Could you check a few things on this model? Use its own coordinates, in mm. A direction names the side the tool comes from. Round coordinates to 2 decimals unless told otherwise and drop trailing zeros. One line per question, with ' | ' between items.
```python
from build123d import *

# Parameters (mm, degrees)
BOSS_EXTRUDE1_DEPTH = 80


with BuildPart() as part:
    # Sketch1 → Boss-Extrude1 (new body)
    with BuildSketch(Plane.XY):
        Polygon((0, 0), (61.257678877, 0), (59.423406602, 35), (58.423406602, 35), (56.851173223, 5), (55.851173223, 5), (54.278939845, 35), (53.278939845, 35), (51.706706466, 5), (50.706706466, 5), (49.134473088, 35), (48.134473088, 35), (46.562239709, 5), (45.562239709, 5), (43.990006331, 35), (42.990006331, 35), (41.417772952, 5), (40.417772952, 5), (38.845539574, 35), (37.845539574, 35), (36.273306195, 5), (35.273306195, 5), (33.701072817, 35), (32.701072817, 35), (31.128839438, 5), (30.128839438, 5), (28.55660606, 35), (27.55660606, 35), (25.984372681, 5), (24.984372681, 5), (23.412139303, 35), (22.412139303, 35), (20.839905924, 5), (19.839905924, 5), (18.267672546, 35), (17.267672546, 35), (15.695439167, 5), (14.695439167, 5), (13.123205789, 35), (12.123205789, 35), (10.55097241, 5), (9.55097241, 5), (7.978739032, 35), (6.978739032, 35), (5.406505653, 5), (4.406505653, 5), (2.834272275, 35), (1.834272275, 35), (0.262038896, 5), align=None)
    extrude(amount=BOSS_EXTRUDE1_DEPTH)


solid = part.part
```
1. I'm going to push flat-ended pins straight in: pin 1 (12 mm diameter, centred on y = 8.5, z = 29, fed in from +X); pin 2 (1.5 mm diameter, centred on x = 54, z = 27, fed in from -Y); pin 3 (0.5 mm diameter, centred on x = 10, z = 55, fed in from +Y); pin 4 (5 mm diameter, centred on y = 14, z = 66, fed in from -X). Where does each tip first touch, or does it pass through?
From the geometry:
pin 1: stops at x = 61.13 | pin 2: stops at y = 0 | pin 3: stops at y = 5 | pin 4: stops at x = 0.6
2. If we mould it in two halves opening along X, with no side actions, what happens to faces 3 (the face through (47.36, 20.21, 39.44)), 4 (the face through (23, 14, 80)), 5 (the face through (60.353, 17.255, 39.44))? For each: pulls with the +X half, pulls with the -X half, needs draft (parallel to the pull), parting line crosses it, or undercut.
From the geometry:
face 3: undercut | face 4: needs draft | face 5: pulls with the +X half
3. I need wall thicknesses on probe 1 along Y at (x, z) = (4.5, 7); probe 2 along X at (y, z) = (2, 12). Which ranges of each line are inside material? Lowest first, please.
From the geometry:
probe 1: y = 0 to 5 | probe 2: x = 0.1 to 61.15
4. I want a section at A-A on y = 6. Count the separate pieces of the cut face and the enclosed holes in it, and give its area (3 significant figures).
From the geometry:
separate pieces: 12 | enclosed holes: 0 | area: 3,880 mm²
5. On a 3-axis mill with a long thin cutter (end or side, diameter ignored), from which of +Z, -Z, +X, -X, +Y, -Y can I reach the whole of each face in a straight line? I mean faces 1 (the face through (16.493, 20.21, 39.44)), 2 (the face through (23, 14, 0)). Say none if no direction works.
From the geometry:
face 1: +Z, -Z, +Y | face 2: -Z, +X, -X, +Y, -Y
